Geometry: final body of the model. Coordinates: model frame, mm. Face numbers are marked on the shaded views. A direction names the side the tool comes from. Give positions to 0.01 mm unless a question says otherwise; leave off trailing zeros. Write each loop counter-clockwise with the first axis right and the second up, starting at its lowest first coordinate (ties: lowest second). Pieces come first, ordered by that corner, then holes. Notation, with made-up numbers: (49.5, 48) -> (54.5, 48) arc R19 ccw to (54.5, 56) -> close; hole circle Ø10 at (-36.75, -1). An arc over 180 degrees is marked (long way). Answer in a Markdown table with one row per item. Add a question column.
Item 1: Access query for the marked faces 4 and 5. Directions: +Z, -Z, +X, -X, +Y, -Y. A direction counts if a zero-diameter tool reaches every point of the face in a straight line with its end or side. Return the directions, or none.
Item 2: First-contact query: P1, Ø5, axis at x = -19.5, y = -2, coming from the +Z side; P2, Ø3, axis at x = 18.5, z = 1.5, coming from the +Y side; P3, Ø0.6, axis at y = -0.5, z = -1.5, coming from the +X side (3 decimals); P4, Ø19.5, axis at x = 2, y = 2, coming from the +Z side. Flat tips, straight axial feed; report the tip coordinate or a pass-through.
Item 3: Draft query along Z for the marked faces 1, 2 and 3. Return one class per face: +Z half, -Z half, draft (parallel to the pull), parting line (faces both ways), or undercut.
Item 4: Section query C-C on x = -30.5. Output: boundary loops of the cut face in (y, z).
Item 5: Material intervals for probe 1 along Y at (x, z) = (0, 10); probe 2 along Y at (x, z) = (0, -21.5); probe 3 along Z at (x, y) = (7, 26.5), sorted ascending. Write a range as from..to.
Item 6: Section query B-B on z = -19. Output: boundary loops of the cut face in (x, y), plus the area to 3 significant figures.
Item 7: Section query A-A on x = 28. Output: boundary loops of the cut face in (y, z), plus the area to 3 significant figures.
```python
from build123d import *

# Parameters (mm, degrees)
SKETCH_R             = 14.5
SKETCH_R_2           = 12.1
PAD_DEPTH            = 14.6
SKETCH001_W          = 30.380329
SKETCH001_H          = 1.5
POCKET_DEPTH         = 97.067871
POLARPATTERN_COUNT   = 3
SKETCH003_R          = 22
PAD001_DEPTH         = 40
SKETCH004_R          = 22
SKETCH004_R_2        = 18.1
PAD002_DEPTH         = 6
PAD003_DEPTH         = 10
SKETCH005_R          = 11
POCKET001_DEPTH      = 50.001
POCKET001_DEPTH_BACK = 14.601
FILLET_R             = 1.5
POCKET002_DEPTH      = 16.601
CHAMFER_SIZE         = 2


with BuildPart() as part:
    # Sketch → Pad (new body)
    with BuildSketch(Plane.XY):
        Circle(SKETCH_R)
        Circle(SKETCH_R_2, mode=Mode.SUBTRACT)
    extrude(amount=PAD_DEPTH)

    # Sketch001 → Pocket (cut, through all)
    with BuildSketch(Plane.XY.offset(4.6)):
        with Locations((15.190164, 0)):
            Rectangle(SKETCH001_W, SKETCH001_H)
    pocket = extrude(amount=POCKET_DEPTH, mode=Mode.SUBTRACT)

    # PolarPattern: Pocket ×3 about axis
    polarpattern_axis = Axis((0, 0, 4.6), (0, 0, 1))
    for i in range(1, POLARPATTERN_COUNT):
        add(pocket.rotate(polarpattern_axis, i * 360 / POLARPATTERN_COUNT), mode=Mode.SUBTRACT)

    # Sketch003 → Pad001 (join)
    with BuildSketch(Plane.XY):
        Circle(SKETCH003_R)
    extrude(amount=-PAD001_DEPTH)

    # Sketch004 → Pad002 (join)
    with BuildSketch(Plane.XY):
        Circle(SKETCH004_R)
        Circle(SKETCH004_R_2, mode=Mode.SUBTRACT)
    extrude(amount=PAD002_DEPTH)

    # Sketch002 → Pad003 (join)
    with BuildSketch(Plane.XY.offset(-40)):
        Polygon((20, -34.641016), (34.641016, -20), (40, 0), (34.641016, 20), (20, 34.641016), (0, 40), (-20, 34.641016), (-34.641016, 20), (-40, 0), (-34.641016, -20), (-20, -34.641016), (0, -40), align=None)
    extrude(amount=-PAD003_DEPTH)

    # Sketch005 → Pocket001 (cut, two sides)
    with BuildSketch(Plane.XY) as pocket001_sk:
        Circle(SKETCH005_R)
    extrude(amount=-POCKET001_DEPTH, mode=Mode.SUBTRACT)
    extrude(pocket001_sk.sketch, amount=POCKET001_DEPTH_BACK, mode=Mode.SUBTRACT)

    # Fillet
    fillet_edges = [part.edges().sort_by_distance(p)[0] for p in [
        (-22, 0, 6),
        (-18.1, 0, 6),
    ]]
    fillet(fillet_edges, radius=FILLET_R)

    # Sketch006 → Pocket002 (cut, through all)
    with BuildSketch(Plane.XY.offset(-2)):
        with BuildLine():
            ThreePointArc((17.565, 4.21), (16.150786, 3.624214), (15.565, 2.21))
            Line((15.565, -2.21), (15.565, 2.21))
            ThreePointArc((15.565, -2.21), (16.150786, -3.624214), (17.565, -4.21))
            Line((34.147769, -4.21), (17.565, -4.21))
            ThreePointArc((34.147769, -4.21), (35.561983, -3.624214), (36.147769, -2.21))
            Line((36.147769, 2.21), (36.147769, -2.21))
            ThreePointArc((36.147769, 2.21), (35.561983, 3.624214), (34.147769, 4.21))
            Line((17.565, 4.21), (34.147769, 4.21))
        make_face()
        with BuildLine():
            ThreePointArc((-49.927467, 4.21), (-51.34168, 3.624214), (-51.927467, 2.21))
            Line((-51.927467, -2.21), (-51.927467, 2.21))
            ThreePointArc((-51.927467, -2.21), (-51.34168, -3.624214), (-49.927467, -4.21))
            Line((-17.565, -4.21), (-49.927467, -4.21))
            ThreePointArc((-17.565, -4.21), (-16.150786, -3.624214), (-15.565, -2.21))
            Line((-15.565, 2.21), (-15.565, -2.21))
            ThreePointArc((-15.565, 2.21), (-16.150786, 3.624214), (-17.565, 4.21))
            Line((-49.927467, 4.21), (-17.565, 4.21))
        make_face()
    extrude(amount=POCKET002_DEPTH, mode=Mode.SUBTRACT)

    # Chamfer
    chamfer_edges = [part.edges().sort_by_distance(p)[0] for p in [
        (27.320508, -27.320508, -50),
        (10, -37.320508, -50),
        (37.320508, -10, -50),
        (-10, -37.320508, -50),
        (37.320508, 10, -50),
        (-27.320508, -27.320508, -50),
        (27.320508, 27.320508, -50),
        (-37.320508, -10, -50),
        (10, 37.320508, -50),
        (-37.320508, 10, -50),
        (-10, 37.320508, -50),
        (-27.320508, 27.320508, -50),
        (-11, 0, -50),
        (27.320508, -27.320508, -40),
        (10, -37.320508, -40),
        (37.320508, -10, -40),
        (-10, -37.320508, -40),
        (37.320508, 10, -40),
        (-27.320508, -27.320508, -40),
        (27.320508, 27.320508, -40),
        (-37.320508, -10, -40),
        (10, 37.320508, -40),
        (-37.320508, 10, -40),
        (-10, 37.320508, -40),
        (-27.320508, 27.320508, -40),
        (-22, 0, -40),
    ]]
    chamfer(chamfer_edges, length=CHAMFER_SIZE)


solid = part.part
```
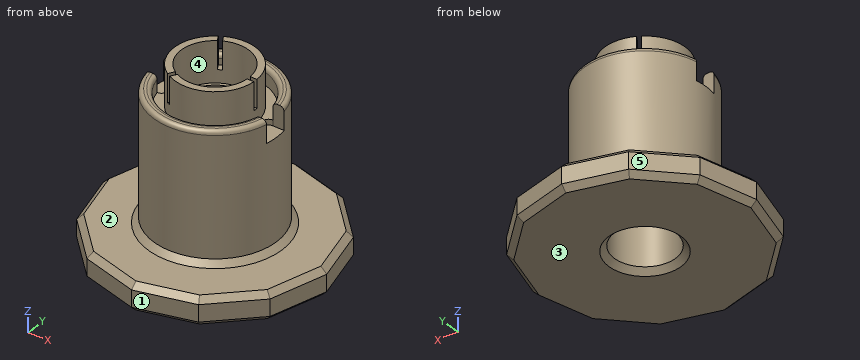
Findings below:
| question | item | result |
|---|---|---|
| 1 | face 4 | +Z |
| 1 | face 5 | +Z, -Z, -X, +Y |
| 2 | P1 | stops at z = 6 |
| 2 | P2 | stops at y = 13.96 |
| 2 | P3 | stops at x = 15.565 |
| 2 | P4 | stops at z = 14.6 |
| 3 | face 1 | draft |
| 3 | face 2 | +Z half |
| 3 | face 3 | -Z half |
| 4 | outline | (-24.14, -48) -> (-21.31, -50) -> (21.31, -50) -> (24.14, -48) -> (24.14, -42) -> (21.31, -40) -> (-21.31, -40) -> (-24.14, -42) -> close |
| 5 | probe 1 | y = -14.5..-12.1, 12.1..14.5 |
| 5 | probe 2 | y = -22..-11, 11..22 |
| 5 | probe 3 | z = -50..-40 |
| 6 | outline | circle Ø44 at (0, 0); hole circle Ø22 at (0, 0) |
| 6 | area | 1,140 mm^2 |
| 7 | outline | (-26.64, -48) -> (-23.81, -50) -> (23.81, -50) -> (26.64, -48) -> (26.64, -42) -> (23.81, -40) -> (-23.81, -40) -> (-26.64, -42) -> close |
| 7 | area | 522 mm^2 |
